Part model, mm, in its own coordinate system. A direction names the side the tool comes from. Round coordinates to 2 decimals unless told otherwise and drop trailing zeros. Order: outer loops, then holes, each group sorted by start corner. A loop starts at its lowest first (then second) coordinate and runs counter-clockwise, first axis right, second up. Notation, with made-up numbers: (-37, 29.25) -> (13, 29.25) arc R26 cw to (13, 66.25) -> close; hole circle Ø7 at (-7, 74). An arc over 180 degrees is marked (long way). Use CSV: the item, a comma, the result in double quotes.
```python
from build123d import *

# Parameters (mm, degrees)
SKETCH1_W           = 31.75
SKETCH1_H           = 31.75
SKETCH1_R           = 1.143
SKETCH1_R_2         = 14.605
BOSS_EXTRUDE1_DEPTH = 1.27
CHAMFER1_SIZE       = 2.54
SKETCH2_W           = 31.75
SKETCH2_H           = 33.02
BOSS_EXTRUDE2_DEPTH = 1.27
SKETCH3_R           = 3.048
CUT_EXTRUDE1_DEPTH  = 1.27
CHAMFER2_SIZE       = 2.54


with BuildPart() as part:
    # Sketch1 → Boss-Extrude1 (new body)
    with BuildSketch(Plane.XY):
        Rectangle(SKETCH1_W, SKETCH1_H)
        with Locations((-11.43, 11.43)):
            Circle(SKETCH1_R, mode=Mode.SUBTRACT)
        with Locations((11.43, 11.43)):
            Circle(SKETCH1_R, mode=Mode.SUBTRACT)
        with Locations((-11.43, -11.43)):
            Circle(SKETCH1_R, mode=Mode.SUBTRACT)
        with Locations((11.43, -11.43)):
            Circle(SKETCH1_R, mode=Mode.SUBTRACT)
        Circle(SKETCH1_R_2, mode=Mode.SUBTRACT)
    extrude(amount=BOSS_EXTRUDE1_DEPTH)

    # Chamfer1
    chamfer1_edges = [part.edges().sort_by_distance(p)[0] for p in [
        (-15.875, 15.875, 0.635),
        (15.875, 15.875, 0.635),
    ]]
    chamfer(chamfer1_edges, length=CHAMFER1_SIZE)

    # Sketch2 → Boss-Extrude2 (add)
    with BuildSketch(Plane.XZ.offset(15.875)):
        with Locations((0, -15.24)):
            Rectangle(SKETCH2_W, SKETCH2_H)
    extrude(amount=BOSS_EXTRUDE2_DEPTH)

    # Sketch3 → Cut-Extrude1 (cut)
    with BuildSketch(Plane(origin=(0, -15.875, 0), x_dir=(1, 0, 0), z_dir=(0, 1, 0))):
        with Locations(Location((0, 15.875, 0), (0, 0, 270))):
            Circle(SKETCH3_R)
    extrude(amount=-CUT_EXTRUDE1_DEPTH, mode=Mode.SUBTRACT)

    # Chamfer2
    chamfer2_edges = [part.edges().sort_by_distance(p)[0] for p in [
        (15.875, -16.51, -31.75),
        (-15.875, -16.51, -31.75),
    ]]
    chamfer(chamfer2_edges, length=CHAMFER2_SIZE)


solid = part.part
```
(1) Cut at C-C, the plane y = -11.43. Give the cut face in (x, z) (3 decimals), then the cut area to 3 significant figures.
Reply:
outline,"(-15.875, 0) -> (-12.573, 0) -> (-12.573, 1.27) -> (-15.875, 1.27) -> close; (-10.287, 0) -> (-9.092, 0) -> (-9.092, 1.27) -> (-10.287, 1.27) -> close; (9.092, 0) -> (10.287, 0) -> (10.287, 1.27) -> (9.092, 1.27) -> close; (12.573, 0) -> (15.875, 0) -> (15.875, 1.27) -> (12.573, 1.27) -> close"
area,"11.4 mm2"
(2) Probe probe 1 along Y at (x, z) = (-11.43, 1) (3 decimals); probe 2 along Y at (x, z) = (15, -3) (3 decimals); probe 3 along Z at (x, y) = (13, 12). List the from-to ranges inside material, lowest first. Write a range as [from, to].
Reply:
probe 1,"[-17.145, -12.573], [-10.287, -9.092], [9.092, 10.287], [12.573, 15.875]"
probe 2,"[-17.145, -15.875]"
probe 3,"[0, 1.27]"
(3) Cut at D-D, the plane x = 11.43. Give the cut face in (y, z) (3 decimals), then the cut area to 3 significant figures.
Reply:
outline,"(-17.145, -31.75) -> (-15.875, -31.75) -> (-15.875, 0) -> (-12.573, 0) -> (-12.573, 1.27) -> (-17.145, 1.27) -> close; (-10.287, 0) -> (-9.092, 0) -> (-9.092, 1.27) -> (-10.287, 1.27) -> close; (9.092, 0) -> (10.287, 0) -> (10.287, 1.27) -> (9.092, 1.27) -> close; (12.573, 0) -> (15.875, 0) -> (15.875, 1.27) -> (12.573, 1.27) -> close"
area,"53.4 mm2"
(4) Which spindle directions (+Z, -Z, +X, -X, +Y, -Y) get a long thin tool onto all of the face, cutting with end or side? Do faces 5 (the face through (-7, -13, 0)), 6 (the face through (11.182, -12.546, 0.626)). Say none if no direction does.
Reply:
face 5,"-Z, +X, -X, +Y"
face 6,"+Z, -Z"
(5) Cut at A-A, the plane x = 0. Give the cut face in (y, z) (3 decimals), then the cut area to 3 significant figures.
Reply:
outline,"(-17.145, -31.75) -> (-15.875, -31.75) -> (-15.875, -18.923) -> (-17.145, -18.923) -> close; (-17.145, -12.827) -> (-15.875, -12.827) -> (-15.875, 0) -> (-14.605, 0) -> (-14.605, 1.27) -> (-17.145, 1.27) -> close; (14.605, 0) -> (15.875, 0) -> (15.875, 1.27) -> (14.605, 1.27) -> close"
area,"37.4 mm2"
(6) Drop flat-ended pins along their axis: P1, Ø12, axis at x = -8, z = -14, coming from the +Y side (3 decimals); P2, Ø3, axis at x = 11.43, y = -11.43, coming from the +Z side; P3, Ø2.5, axis at x = -11.43, y = 11.43, coming from the -Z side. Give the stop position or say it passes through.
Reply:
P1,"y = -15.875"
P2,"z = 1.27"
P3,"z = 0"
(7) Cut at B-B, the plane y = 0. Give the cut face in (x, z) (3 decimals), then the cut area to 3 significant figures.
Reply:
outline,"(-15.875, 0) -> (-14.605, 0) -> (-14.605, 1.27) -> (-15.875, 1.27) -> close; (14.605, 0) -> (15.875, 0) -> (15.875, 1.27) -> (14.605, 1.27) -> close"
area,"3.23 mm2"
(8) Pull direction X, two halves, no side cores. Call faces 1 (the face through (11.281, 12.563, 0.626)), 2 (the face through (14.623, -16.501, -30.462)), 3 (the face through (-11.678, -12.546, 0.626)), 4 (the face through (3.3, -17.145, -15)): released by +X, released by -X, zero draft, split by the parting line, or undercut.
Reply:
face 1,"undercut"
face 2,"released by +X"
face 3,"undercut"
face 4,"zero draft"
